Design review of the part built by this model. Coordinates are the model's own, in mm. A direction names the side the tool comes from. Give positions to 0.01 mm unless a question says otherwise; leave off trailing zeros. Loops run counter-clockwise (first coordinate to the right, second up) from the corner with the lowest first, then second, coordinate; pieces in that order, holes last. Notation, with made-up numbers: (62, 87) - (117, 87) arc R22 ccw to (117, 114) - close; hole circle Ø9 at (41.25, 46). An arc over 180 degrees is marked (long way). Write each question's results on one line, items separated by ' | '.
Autodesk Inventor part; units mm, degrees
ref_plane "YZ Plane" through (0, 0, 0) normal (1, 0, 0) x (0, 1, 0)
ref_plane "XZ Plane" through (0, 0, 0) normal (0, 1, 0) x (-1, 0, 0)
ref_plane "XY Plane" through (0, 0, 0) normal (0, 0, 1) x (1, 0, 0)
sketch "Sketch1" plane through (0, 0, 0) normal (0, 0, 1) x (1, 0, 0)
  line L0 (0, 0) -> (38.1, 0)
  line L1 (38.1, 0) -> (38.1, 253.0348)
  arc A0 (38.1, 507.0348) -> (38.1, 253.0348) centre (666.75, 380.0348) ccw
  line L2 (38.1, 507.0348) -> (38.1, 608.6348)
  line L3 (38.1, 608.6348) -> (0, 608.6348)
  line L4 (0, 608.6348) -> (0, 0)
  circle A1 centre (31.75, 151.4348) radius 3.3655
  circle A2 centre (31.75, 34.671) radius 3.3655
  circle A3 centre (12.7, 12.7) radius 3.3655
  circle A4 centre (12.7, 342.9) radius 3.3655
  circle A5 centre (12.7, 595.9348) radius 3.3655
  circle A6 centre (31.75, 12.7) radius 3.3655
  circle A7 centre (31.75, 253.0348) radius 3.3655
  circle A8 centre (31.75, 507.0348) radius 3.3655
  circle A9 centre (31.75, 595.9348) radius 3.3655
  line L5 (0, 557.8348) -> (0, 608.6348)
  line L6 (0, 50.8) -> (0, 0)
  line L7 (12.7, 342.9) -> (0, 304.3174) construction
  line L8 (0, 317.5) -> (0, 368.3)
  line L9 (0, 129.921) -> (12.7, 129.921) construction
  circle A10 centre (12.7, 129.921) radius 3.3655
  circle A11 centre (12.7, 174.371) radius 3.3655
  line L10 (9.3413, 197.482) -> (9.3413, 204.213)
  line L11 (16.0611, 204.488) -> (16.0611, 197.3435)
  arc A12 (16.0611, 204.488) -> (9.3413, 204.213) centre (12.6956, 204.488) ccw
  arc A13 (9.3413, 197.482) -> (16.0611, 197.3435) centre (12.6974, 197.231) ccw
  circle A14 centre (12.7, 217.188) radius 3.3655
  dimension "d0" = 38.1
  dimension "d2" = 101.6
  dimension "d4" = 457.2
  dimension "d5" = 101.6
  dimension "d6" = 666.75
  dimension "d7" = 641.35
  dimension "d9" = 116.7638
  dimension "d10" = 6.35
  dimension "d11" = 6.35
  dimension "d13" = 12.7
  dimension "d14" = 12.7
  dimension "d16" = 12.7
  dimension "d17" = 342.9
  dimension "d19" = 12.7
  dimension "d20" = 12.7
  dimension "d22" = 6.35
  dimension "d24" = 6.35
  dimension "d25" = 6.731
  dimension "d26" = 6.35
  dimension "hole" = 6.731
  dimension "d28" = 6.35
  dimension "d45" = 12.7
  dimension "d47" = 12.7
  dimension "d54" = 6.731
  dimension "d55" = 3.3655
  dimension "d56" = 3.3655
  dimension "d58" = 6.731
  dimension "d59" = 12.7
  dimension "d68" = 18.22
  dimension "d69" = 90
  dimension "d70" = 90
  dimension "d71" = 22.0389
  dimension "d72" = 28.7587
  dimension "d73" = 478.7138
  dimension "d74" = 6.35
  dimension "d75" = 6.35
  dimension "d76" = 595.9348
  dimension "d77" = 404.1468
  dimension "d78" = 411.2913
  dimension "d79" = 25.4
  dimension "d80" = 25.4
  dimension "d81" = 434.2638
  dimension "d82" = 50.8
  dimension "d83" = 240.3348
  dimension "d84" = 291.1348
  dimension "d85" = 557.8348
extrude "Plate4" add sketch "Sketch1" along normal blind 3.048
sketch "Sketch5" plane through (0, 0, 3.048) normal (0, 0, 1) x (1, 0, 0)
  line L0 (38.1, 0) -> (38.1, 253.0348)
  line L1 (0, 0) -> (38.1, 0)
  line L2 (38.1, 0) -> (38.1, 25.4)
  line L3 (38.1, 25.4) -> (0, 25.4)
  line L4 (0, 25.4) -> (0, 0)
  dimension "d96" = 25.4
extrude "Cut1" cut sketch "Sketch5" against normal blind 3.048
sketch "Sketch7" plane through (0, 25.4, 3.048) normal (-1, 0, 0) x (0, -1, 0)
  line L0 (-583.2348, 0) -> (0, 0)
  line L1 (0, 0) -> (0, 22.352)
  line L2 (0, 22.352) -> (-583.2348, 22.352)
  line L3 (-583.2348, 22.352) -> (-583.2348, 0)
edge flange "Flange3" height 25.4 angle 90 thickness 3.048 bend radius 3.048 thickness toward (-1, 0, 0) relief tear relief width 3.048 relief depth 1.524 edges at (0, 317.0174, 3.048) wall of the first edge with corners at (0, 608.6348, 3.048) (0, 25.4, 3.048) (0, 25.4, 25.4) (0, 608.6348, 25.4)
bend "Bend3"
corner "Corner3"
equation "\"d25\" = hole"
equation "\"d97\" = Thickness"
equation "\"d109\" = BendReliefWidth"
equation "\"d110\" = BendReliefDepth"
equation "\"d111\" = MinimumRemnant"
equation "\"d112\" = BendRadius"
equation "\"d115\" = BendRadius"
equation "\"d116\" = CornerReliefSize"
equation "\"d117\" = GapSize"
equation "\"d118\" = JacobiRadiusSize"
equation "\"BendRadius\" = Thickness"
equation "\"BendReliefWidth\" = Thickness"
equation "\"BendReliefDepth\" = 0.5 * Thickness"
equation "\"CornerReliefSize\" = 4 * Thickness"
equation "\"MinimumRemnant\" = 2 * Thickness"
equation "\"TransitionRadius\" = BendRadius"
equation "\"JacobiRadiusSize\" = BendRadius"
equation "\"GapSize\" = Thickness"
equation "\"d29\" = BendRadius"
equation "\"d32\" = BendRadius"
equation "\"d38\" = BendRadius"
equation "\"d60\" = BendRadius"
properties part number "clawRTOP-v2"
Item 1: Tool access review of faces 1 (the face through (0, 313, 16)), 2 (the face through (20, 321, 0)): name each direction out of +Z, -Z, +X, -X, +Y, -Y from which nothing blocks a thin tool from reaching the whole face with its end or side.
Output values:
face 1: +Z, +X, +Y, -Y | face 2: -Z, +X, -X, +Y, -Y
Item 2: We need section B-B on z = 16.25. Give the boundary of the cut face in (x, y), then the cut area to 3 significant figures.
Output values:
outline: (-3.05, 25.4) - (0, 25.4) - (0, 608.63) - (-3.05, 608.63) - close | area: 1,780 mm²
Item 3: We need section A-A on y = 330.5. Give the boundary of the cut face in (x, z).
Output values:
outline: (-3.05, 6.1) arc R6.1 ccw to (3.05, 0) - (27.32, 0) - (27.32, 3.05) - (3.05, 3.05) arc R3.05 cw to (0, 6.1) - (0, 25.4) - (-3.05, 25.4) - close
Item 4: Wall thickness on probe 1 along X at (y, z) = (342.9, 0.9); probe 2 along Z at (x, y) = (21, 472); probe 3 along X at (y, z) = (197, 8): over which ranges is each line inside the solid? List them lowest first.
Output values:
probe 1: x = -0.14 to 9.33, 16.07 to 26.48 | probe 2: z = 0 to 3.05 | probe 3: x = -3.05 to 0
Item 5: Draft analysis for pull direction Y (two halves, no side actions). For faces 3 (the face through (10, 25.4, 2)), 4 (the face through (-3.048, 313, 16)), 5 (the face through (25.402, 378.245, 1.503)), state which applies: +Y half, -Y half, draft (parallel to the pull), parting line (faces both ways), or undercut.
Output values:
face 3: -Y half | face 4: draft | face 5: undercut
Item 6: Clearance check with flat-ended pins moving along their axes: P1, Ø7.5, axis at x = 31.75, y = 507.03, coming from the +Z side; P2, Ø3.5, axis at y = 200.5, z = 1, coming from the -X side; P3, Ø5.5, axis at x = 31.75, y = 151.43, coming from the +Z side; P4, Ø2, axis at y = 276.5, z = 17, coming from the +X side. State where each tip first meets the part, or that it passes through.
Output values:
P1: stops at z = 3.05 | P2: stops at x = -2.05 | P3: passes through | P4: stops at x = 0
